Source: CAD feature listing. Evaluate the final solid. Frame: model axes, mm. A direction names the side the tool comes from. Give positions to 0.01 mm unless a question says otherwise; leave off trailing zeros. Loops run counter-clockwise (first coordinate to the right, second up) from the corner with the lowest first, then second, coordinate; pieces in that order, holes last. Notation, with made-up numbers: (20, 6) -> (44, 6) arc R26 cw to (44, 38) -> close; hole circle Ø8 at (86, 68.25). An arc over 180 degrees is marked (long way). Put each result on its own line as item: value.
```python
from build123d import *

# Parameters (mm, degrees)
SKETCH1_W            = 150
SKETCH1_H            = 90
BOSS_EXTRUDE1_DEPTH  = 135
SKETCH2_W            = 140
SKETCH2_H            = 60
CUT_EXTRUDE1_DEPTH   = 135
SKETCH3_W            = 3
SKETCH3_H            = 45
BOSS_EXTRUDE2_DEPTH  = 17
SKETCH4_W            = 22
SKETCH4_H            = 5
BOSS_EXTRUDE3_DEPTH  = 7
MIRROR2_OUTLINE_W    = 7
MIRROR2_OUTLINE_H    = 22
MIRROR2_DEPTH        = 5
SKETCH5_W            = 10
SKETCH5_H            = 10
CUT_EXTRUDE3_DEPTH   = 220.406016326
SKETCH6_W            = 56
SKETCH6_H            = 18
BOSS_EXTRUDE4_DEPTH  = 1.5
SKETCH7_W            = 18
SKETCH7_H            = 90
BOSS_EXTRUDE5_DEPTH  = 3
FILLET1_R            = 9
BOSS_EXTRUDE6_DEPTH  = 1.5
SKETCH11_W           = 60
SKETCH11_H           = 18
BOSS_EXTRUDE7_DEPTH  = 3
FILLET2_R            = 9
BOSS_EXTRUDE8_DEPTH  = 1.5
BOSS_EXTRUDE9_DEPTH  = 18
SKETCH15_W           = 25
SKETCH15_H           = 18
BOSS_EXTRUDE10_DEPTH = 1.5
FILLET3_R            = 6
SKETCH16_W           = 21
SKETCH16_H           = 3
BOSS_EXTRUDE11_DEPTH = 1.5
SKETCH17_W           = 3.8
SKETCH17_H           = 4
SKETCH17_H_2         = 3
SKETCH17_W_2         = 2
SKETCH17_H_3         = 15
BOSS_EXTRUDE13_DEPTH = 1.5
SKETCH18_W           = 31
SKETCH18_H           = 18
BOSS_EXTRUDE14_DEPTH = 1.5
SKETCH19_W           = 22
SKETCH19_H           = 5
CUT_EXTRUDE4_DEPTH   = 14
SKETCH20_W           = 22
SKETCH20_H           = 5
CUT_EXTRUDE5_DEPTH   = 7
SKETCH21_W           = 22
SKETCH21_H           = 1.2
BOSS_EXTRUDE15_DEPTH = 5


# Read off the part's stored shape, not the designer's step: Mirror2
with BuildPart() as part:
    # Sketch1 → Boss-Extrude1 (new body)
    with BuildSketch(Plane(origin=(0, 0, 0), x_dir=(1, 0, 0), z_dir=(0, 1, 0))):
        Rectangle(SKETCH1_W, SKETCH1_H)
    extrude(amount=BOSS_EXTRUDE1_DEPTH)

    # Sketch2 → Cut-Extrude1 (cut)
    with BuildSketch(Plane.XY.offset(45)):
        with Locations((0, 35)):
            Rectangle(SKETCH2_W, SKETCH2_H)
        with Locations((0, 100)):
            Rectangle(SKETCH2_W, SKETCH2_H)
    extrude(amount=-CUT_EXTRUDE1_DEPTH, mode=Mode.SUBTRACT)

    # Sketch3 → Boss-Extrude2 (add)
    with BuildSketch(Plane(origin=(75, 0, 0), x_dir=(0, 0, -1), z_dir=(1, 0, 0))):
        with Locations((12.5, 22.5)):
            Rectangle(SKETCH3_W, SKETCH3_H)
        with Locations((-12.5, 22.5)):
            Rectangle(SKETCH3_W, SKETCH3_H)
    boss_extrude2 = extrude(amount=BOSS_EXTRUDE2_DEPTH)

    # Mirror1: Boss-Extrude2 across plane
    add(boss_extrude2.mirror(Plane(origin=(0, 0, 0), x_dir=(0, 0, 1), z_dir=(1, 0, 0))))

    # Sketch4 → Boss-Extrude3 (add)
    with BuildSketch(Plane.ZY.offset(75)):
        with Locations((0, 2.5)):
            Rectangle(SKETCH4_W, SKETCH4_H)
    extrude(amount=BOSS_EXTRUDE3_DEPTH)

    # Mirror2 outline → Mirror2 (add)
    with BuildSketch(Plane(origin=(0, 0, 0), x_dir=(1, 0, 0), z_dir=(0, 1, 0))):
        with Locations((-85.5, 0)):
            Rectangle(MIRROR2_OUTLINE_W, MIRROR2_OUTLINE_H)
        with Locations((78.5, 0)):
            Rectangle(MIRROR2_OUTLINE_W, MIRROR2_OUTLINE_H)
    extrude(amount=MIRROR2_DEPTH)

    # Sketch5 → Cut-Extrude3 (cut, through all)
    with BuildSketch(Plane.ZY.offset(75)):
        with Locations((0, 10)):
            Rectangle(SKETCH5_W, SKETCH5_H)
    extrude(amount=-CUT_EXTRUDE3_DEPTH, mode=Mode.SUBTRACT)

    # Sketch6 → Boss-Extrude4 (add)
    with BuildSketch(Plane(origin=(0, 135, 0), x_dir=(1, 0, 0), z_dir=(0, 1, 0))):
        with Locations((0, -4)):
            Rectangle(SKETCH6_W, SKETCH6_H)
    extrude(amount=BOSS_EXTRUDE4_DEPTH)

    # Sketch7 → Boss-Extrude5 (add)
    with BuildSketch(Plane(origin=(0, 5, 0), x_dir=(1, 0, 0), z_dir=(0, 1, 0))):
        with Locations((45, 0)):
            Rectangle(SKETCH7_W, SKETCH7_H)
        with Locations((-45, 0)):
            Rectangle(SKETCH7_W, SKETCH7_H)
    extrude(amount=BOSS_EXTRUDE5_DEPTH)

    # Fillet1
    fillet1_edges = [part.edges().sort_by_distance(p)[0] for p in [
        (36, 6.5, 45),
        (54, 6.5, 45),
        (-36, 6.5, 45),
        (-54, 6.5, 45),
        (-54, 6.5, -45),
        (-36, 6.5, -45),
        (54, 6.5, -45),
        (36, 6.5, -45),
    ]]
    fillet(fillet1_edges, radius=FILLET1_R - 0.0001)  # a hair under: the kernel refuses the full size

    # Sketch10 → Boss-Extrude6 (add)
    with BuildSketch(Plane(origin=(0, 8, 0), x_dir=(1, 0, 0), z_dir=(0, 1, 0))):
        with BuildLine():
            Line((-45, 45), (-45, -45))
            ThreePointArc((-45, -45), (-51.363961031, -42.363961031), (-54, -36))
            Line((-54, -36), (-54, 36))
            ThreePointArc((-54, 36), (-51.363961031, 42.363961031), (-45, 45))
        make_face()
        with BuildLine():
            Line((45, 45), (45, -45))
            ThreePointArc((45, -45), (51.363961031, -42.363961031), (54, -36))
            Line((54, -36), (54, 36))
            ThreePointArc((54, 36), (51.363961031, 42.363961031), (45, 45))
        make_face()
    extrude(amount=BOSS_EXTRUDE6_DEPTH)

    # Sketch11 → Boss-Extrude7 (add)
    with BuildSketch(Plane(origin=(0, 5, 0), x_dir=(1, 0, 0), z_dir=(0, 1, 0))):
        with Locations((0, 35)):
            Rectangle(SKETCH11_W, SKETCH11_H)
        with Locations((0, -35)):
            Rectangle(SKETCH11_W, SKETCH11_H)
    extrude(amount=BOSS_EXTRUDE7_DEPTH)

    # Fillet2
    fillet2_edges = [part.edges().sort_by_distance(p)[0] for p in [
        (30, 6.5, -26),
        (30, 6.5, -44),
        (-30, 6.5, 26),
        (-30, 6.5, 44),
    ]]
    fillet(fillet2_edges, radius=FILLET2_R - 0.0001)  # a hair under: the kernel refuses the full size

    # Sketch13 → Boss-Extrude8 (add)
    with BuildSketch(Plane(origin=(0, 8, 0), x_dir=(1, 0, 0), z_dir=(0, 1, 0))):
        with BuildLine():
            Line((21, 44), (-30, 44))
            Line((-30, 44), (-30, 35))
            Line((-30, 35), (30, 35))
            ThreePointArc((30, 35), (27.363961031, 41.363961031), (21, 44))
        make_face()
        with BuildLine():
            Line((-21, -44), (30, -44))
            Line((30, -44), (30, -35))
            Line((30, -35), (-30, -35))
            ThreePointArc((-30, -35), (-27.363961031, -41.363961031), (-21, -44))
        make_face()
    extrude(amount=BOSS_EXTRUDE8_DEPTH)

    # Sketch14 → Boss-Extrude9 (add)
    with BuildSketch(Plane(origin=(0, 70, 0), x_dir=(1, 0, 0), z_dir=(0, 1, 0))):
        Polygon((-47.5, -30), (37.5, -30), (37.5, -20), (-37.5, -20), (-37.5, 20), (37.5, 20), (37.5, 30), (-47.5, 30), align=None)
    extrude(amount=BOSS_EXTRUDE9_DEPTH)

    # Sketch15 → Boss-Extrude10 (add)
    with BuildSketch(Plane(origin=(0, 88, 0), x_dir=(1, 0, 0), z_dir=(0, 1, 0))):
        with Locations((0, -29)):
            Rectangle(SKETCH15_W, SKETCH15_H)
        with Locations((0, 29)):
            Rectangle(SKETCH15_W, SKETCH15_H)
    extrude(amount=BOSS_EXTRUDE10_DEPTH)

    # Fillet3
    fillet3_edges = [part.edges().sort_by_distance(p)[0] for p in [
        (-12.5, 88.75, 20),
        (12.5, 88.75, 20),
        (-12.5, 88.75, -20),
        (12.5, 88.75, -20),
    ]]
    fillet(fillet3_edges, radius=FILLET3_R)

    # Sketch16 → Boss-Extrude11 (add)
    with BuildSketch(Plane(origin=(0, 136.5, 0), x_dir=(1, 0, 0), z_dir=(0, 1, 0))):
        Polygon((-10, 5), (-28, 5), (-28, -13), (-10, -13), (-10, -10), align=None)
        with Locations((0.5, -11.5)):
            Rectangle(SKETCH16_W, SKETCH16_H)
        Polygon((28, 5), (11, 5), (11, -10), (11, -13), (28, -13), align=None)
    extrude(amount=BOSS_EXTRUDE11_DEPTH)

    # Sketch17 → Boss-Extrude13 (add)
    with BuildSketch(Plane(origin=(0, 138, 0), x_dir=(1, 0, 0), z_dir=(0, 1, 0))):
        Polygon((10.8, -6), (10.8, -10), (11, -10), (11, 5), (10.8, 5), align=None)
        Polygon((10.8, -10), (10.8, -13), (28, -13), (28, 5), (11, 5), (11, -10), align=None)
        with Locations((8.9, -8)):
            Rectangle(SKETCH17_W, SKETCH17_H)
        with Locations((8.9, -11.5)):
            Rectangle(SKETCH17_W, SKETCH17_H_2)
        Polygon((-10, 5), (-28, 5), (-28, -13), (-8, -13), (-8, -10), (-10, -10), align=None)
        with Locations((-9, -2.5)):
            Rectangle(SKETCH17_W_2, SKETCH17_H_3)
    extrude(amount=BOSS_EXTRUDE13_DEPTH)

    # Sketch18 → Boss-Extrude14 (add)
    with BuildSketch(Plane.ZY.offset(75)):
        with Locations((29.5, 9)):
            Rectangle(SKETCH18_W, SKETCH18_H)
        with Locations((-29.5, 9)):
            Rectangle(SKETCH18_W, SKETCH18_H)
    boss_extrude14 = extrude(amount=BOSS_EXTRUDE14_DEPTH)

    # Mirror3: Boss-Extrude14 across plane
    add(boss_extrude14.mirror(Plane(origin=(0, 0, 0), x_dir=(0, 0, 1), z_dir=(1, 0, 0))))

    # Sketch19 → Cut-Extrude4 (cut)
    with BuildSketch(Plane.ZY.offset(89)):
        with Locations((0, 2.5)):
            Rectangle(SKETCH19_W, SKETCH19_H)
    extrude(amount=-CUT_EXTRUDE4_DEPTH, mode=Mode.SUBTRACT)

    # Sketch20 → Cut-Extrude5 (cut)
    with BuildSketch(Plane(origin=(82, 0, 0), x_dir=(0, 0, -1), z_dir=(1, 0, 0))):
        with Locations((0, 2.5)):
            Rectangle(SKETCH20_W, SKETCH20_H)
    extrude(amount=-CUT_EXTRUDE5_DEPTH, mode=Mode.SUBTRACT)

    # Sketch21 → Boss-Extrude15 (add)
    with BuildSketch(Plane(origin=(75, 0, 0), x_dir=(0, 0, -1), z_dir=(1, 0, 0))):
        with Locations((0, 0.6)):
            Rectangle(SKETCH21_W, SKETCH21_H)
    boss_extrude15 = extrude(amount=BOSS_EXTRUDE15_DEPTH)

    # Mirror4: Boss-Extrude15 across plane
    add(boss_extrude15.mirror(Plane(origin=(0, 0, 0), x_dir=(0, 0, 1), z_dir=(1, 0, 0))))


solid = part.part
```
(1) Section A-A on y = 76. Return loops of the section in (x, z).
Calculated:
outline: (-75, -45) -> (-70, -45) -> (-70, 45) -> (-75, 45) -> close; (-47.5, -30) -> (37.5, -30) -> (37.5, -20) -> (-37.5, -20) -> (-37.5, 20) -> (37.5, 20) -> (37.5, 30) -> (-47.5, 30) -> close; (70, -45) -> (75, -45) -> (75, 45) -> (70, 45) -> close
(2) Section B-B on y = 112. Return loops of the section in (x, z), then the cut area to 3 significant figures.
Calculated:
outline: (-75, -45) -> (-70, -45) -> (-70, 45) -> (-75, 45) -> close; (70, -45) -> (75, -45) -> (75, 45) -> (70, 45) -> close
area: 900 mm²
(3) Reachability of faces 1 (the flat face through (0, 89.5, -29)), 2 (the flat face through (-1, 5, -1)), 3 (the cylindrical face through (-27.434, 8.74, 41.294)), 4 (the cylindrical face through (-38.706, 6.521, -42.434)) from +Z, -Z, +X, -X, +Y, -Y: full face, straight path, thin tool, end or side. Return the list, or none.
Calculated:
face 1: +Z, -Z
face 2: none
face 3: +Z
face 4: -Z
(4) Section C-C on z = 16.5. Give the number of separate pieces and of enclosed holes in the cut face, then the cut area to 3 significant figures.
Calculated:
separate pieces: 1
enclosed holes: 2
area: 3,820 mm²
(5) Draft query along X for faces 5 (the flat face through (-18, 139.5, 4)), 6 (the cylindrical face through (-51.294, 6.521, 42.434)). Return one class per face: released by +X, released by -X, zero draft, split by the parting line, or undercut.
Calculated:
face 5: zero draft
face 6: undercut
(6) First-contact query: P1, Ø2, axis at y = 85, z = 23.5, coming from the -X side; P2, Ø1.6, axis at x = -10.5, y = 9, coming from the -Z side; P3, Ø2.5, axis at x = 13, z = 32, coming from the +Y side. Flat tips, straight axial feed; report the tip coordinate or a pass-through.
Calculated:
P1: stops at x = -75
P2: stops at z = -44
P3: stops at y = 135
(7) Line query: probe 1 along Y at (x, z) = (-53, -40.5); probe 2 along Y at (x, z) = (24, -3); probe 3 along X at (y, z) = (112, -17.5). Output: solid intervals per line, ascending. Write a range as from..to.
Calculated:
probe 1: y = 0..5, 65..70, 130..135
probe 2: y = 0..5, 65..70, 130..139.5
probe 3: x = -75..-70, 70..75
